from build123d import *

# Parameters (mm, degrees)
F1_DEPTH      = 12
F2_W          = 150
F2_H          = 12
F3_DEPTH      = 90
F4_SIZE2      = 35
F4_SIZE       = 35
F5_W          = 15
F5_H          = 33
F6_DEPTH      = 55
F8_DEPTH      = 60
F8_DEPTH_BACK = 60


with BuildPart() as f1:
    # F0 (on Top) → F1 (new body)
    with BuildSketch(Plane.XY):
        Polygon((75, 20.5), (-75, 20.5), (-75, -7.5), (0, -32.5), (75, -7.5), align=None)
    extrude(amount=F1_DEPTH)

    # F2 (on Top) → F3 (join)
    with BuildSketch(Plane.XY):
        with Locations((0, 26.5)):
            Rectangle(F2_W, F2_H)
    extrude(amount=F3_DEPTH)

    # F4
    f4_edges = [f1.edges().sort_by_distance(p)[0] for p in [
        (-75, 26.5, 90),
        (75, 26.5, 90),
    ]]
    chamfer(f4_edges, length=F4_SIZE, length2=F4_SIZE2)

    # F5 (on Top) → F6 (join)
    with BuildSketch(Plane.XY):
        with Locations((-52.5, 4)):
            Rectangle(F5_W, F5_H)
        with Locations((52.5, 4)):
            Rectangle(F5_W, F5_H)
    extrude(amount=F6_DEPTH)

    # F7 (on Right) → F8 (cut, two sides)
    with BuildSketch(Plane.YZ) as f8_sk:
        Polygon((-12.5, 12), (20.5, 55), (-12.5, 55), align=None)
    extrude(amount=-F8_DEPTH, mode=Mode.SUBTRACT)
    extrude(f8_sk.sketch, amount=F8_DEPTH_BACK, mode=Mode.SUBTRACT)


solid = f1.part
Model file for the job. Use its own axes, mm. A direction names the side the tool comes from. Round coordinates to 2 decimals unless told otherwise and drop trailing zeros. Order: outer loops, then holes, each group sorted by start corner. A loop starts at its lowest first (then second) coordinate and runs counter-clockwise, first axis right, second up.
(1) 3-axis set-ups, long thin cutter, end or side, ignore diameter. For faces 5 (the face through (-45, 11, 24)), 6 (the face through (-68, 4, 12)), 7 (the face through (67, 4, 12)), 8 (the face through (-1, 8, 0)): which of +Z, -Z, +X, -X, +Y, -Y reach the whole face in a straight line?
(2) Band-saw the part on D-D (z = 71). List the corners of the cut face in (x, y), then the cut area to 3 significant figures.
(3) Pin check, flat tips, straight feed: pin 1 (1 mm diameter, centred on x = 52, z = 18.5, fed in from -Y); pin 2 (7.5 mm diameter, centred on x = 70, y = 6.5, fed in from +Z); pin 3 (23.5 mm diameter, centred on x = -6, z = 52, fed in from -Y). Stop position of each tip, or through.
(4) Band-saw the part on A-A (y = 25). List the corners of the cut face in (x, z).
(5) Band-saw the part on C-C (z = 43). List the corners of the cut face in (x, y).
(6) Pull direction X, two halves, no side cores. Call faces 1 (the face through (-52.4, 3.77, 33.2)), 2 (the face through (-1, 20.5, 50)), 3 (the face through (-75, 21, 21)), 4 (the face through (45, 11, 24)): released by +X, released by -X, zero draft, split by the parting line, or undercut.
(7) Band-saw the part on B-B (x = -51). List the corners of the cut face in (y, z), then the cut area to 3 significant figures.
(8) Drill centre lines: line 1 (Z direction, x = 28.5, y = 12); line 2 (Y direction, x = -26.5, z = 55.5); line 3 (Y direction, x = 49.5, z = 7). Where is each one in solid material? Low to high.
Verdict:
1. face 5: +Z, -Y
1. face 6: +Z, -X, -Y
1. face 7: +Z, +X, -Y
1. face 8: -Z, +X, -X, +Y, -Y
2. outline: (-59, 20.5) - (59, 20.5) - (59, 32.5) - (-59, 32.5) - close
2. area: 1,420 mm2
3. pin 1: stops at y = -7.9
3. pin 2: stops at z = 12
3. pin 3: stops at y = 20.5
4. outline: (-75, 0) - (75, 0) - (75, 55) - (40, 90) - (-40, 90) - (-75, 55) - close
5. outline: (-75, 20.5) - (-60, 20.5) - (-60, 11.29) - (-45, 11.29) - (-45, 20.5) - (45, 20.5) - (45, 11.29) - (60, 11.29) - (60, 20.5) - (75, 20.5) - (75, 32.5) - (-75, 32.5) - close
6. face 1: zero draft
6. face 2: undercut
6. face 3: released by -X
6. face 4: undercut
7. outline: (-15.5, 0) - (32.5, 0) - (32.5, 79) - (20.5, 79) - (20.5, 55) - (-12.5, 12) - (-15.5, 12) - close
7. area: 2,090 mm2
8. line 1: z = 0 to 12
8. line 2: y = 20.5 to 32.5
8. line 3: y = -16 to 32.5
